Design review of the part shown in the three views and the two pictorial views. Dimensions are in mm from the part's minimum x, y and z. A direction names the side the tool comes from. Coordinates: 2 decimals unless noted, no trailing zeros. Loops run counter-clockwise (first coordinate to the right, second up) from the corner with the lowest first, then second, coordinate; pieces in that order, holes last. Notation, with made-up numbers: (-20.75, 46.5) -> (12.25, 46.5) arc R21 cw to (12.25, 68.5) -> close; hole circle Ø10 at (-15, 43.25). An arc over 180 degrees is marked (long way). Answer in a Markdown table with one row per item.
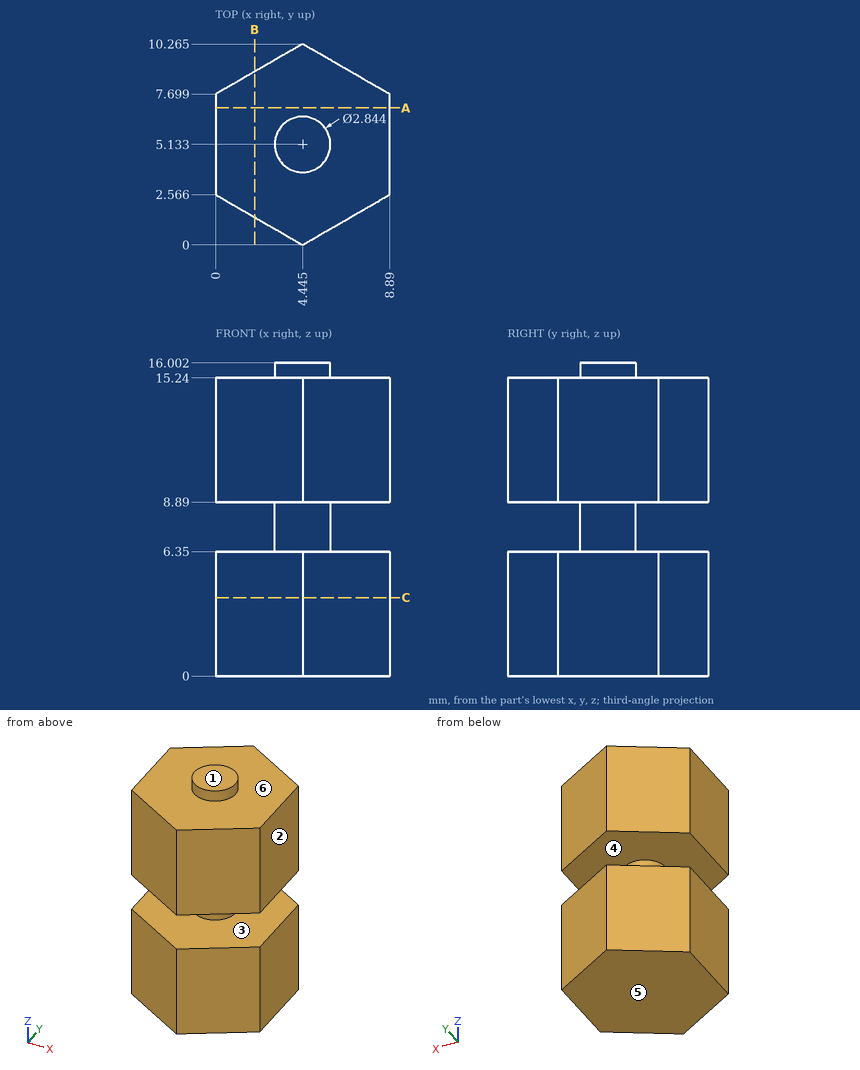
(1) Take a section at C-C on z = 4. Give the boundary of the cut face in (x, y) (1 decimal).
Evaluation:
| item | result |
|---|---|
| outline | (0, 2.6) -> (4.4, 0) -> (8.9, 2.6) -> (8.9, 7.7) -> (4.4, 10.3) -> (0, 7.7) -> close |
(2) Tool access review of the marked faces 5 and 6: name each direction out of +Z, -Z, +X, -X, +Y, -Y from which nothing blocks a thin tool from reaching the whole face with its end or side.
Evaluation:
| item | result |
|---|---|
| face 5 | -Z, +X, -X, +Y, -Y |
| face 6 | +Z |
(3) Take a section at B-B on x = 2. Give the boundary of the cut face in (y, z).
Evaluation:
| item | result |
|---|---|
| outline | (1.41, 0) -> (8.85, 0) -> (8.85, 6.35) -> (1.41, 6.35) -> close; (1.41, 8.89) -> (8.85, 8.89) -> (8.85, 15.24) -> (1.41, 15.24) -> close |
(4) To check wall thickness, follow probe 1 along Z at (x, y) = (7.5, 2.75); probe 2 along X at (y, z) = (2, 10.25); probe 3 along Y at (x, z) = (5.5, 8.5) (1 decimal). State the ranges of each line that lie inside material, in increasing order.
Evaluation:
| item | result |
|---|---|
| probe 1 | z = 0 to 6.35, 8.89 to 15.24 |
| probe 2 | x = 0.98 to 7.91 |
| probe 3 | y = 4.2 to 6.1 |
(5) Take a section at A-A on y = 7. Give the boundary of the cut face in (x, z).
Evaluation:
| item | result |
|---|---|
| outline | (0, 0) -> (8.89, 0) -> (8.89, 6.35) -> (0, 6.35) -> close; (0, 8.89) -> (8.89, 8.89) -> (8.89, 15.24) -> (0, 15.24) -> close |
(6) Draft analysis for pull direction Z (two halves, no side actions). For the marked faces 1, 2, 3 and 4, state which applies: pulls with the +Z half, pulls with the -Z half, needs draft (parallel to the pull), parting line crosses it, or undercut.
Evaluation:
| item | result |
|---|---|
| face 1 | pulls with the +Z half |
| face 2 | needs draft |
| face 3 | undercut |
| face 4 | undercut |
